Check sheet for the modelled part. Datum: model origin and axes. Units: mm. A direction names the side the tool comes from. Give positions to 0.01 mm unless a question says otherwise; leave off trailing zeros. Order: outer loops, then holes, each group sorted by start corner. A loop starts at its lowest first (then second) coordinate and runs counter-clockwise, first axis right, second up. Notation, with made-up numbers: M 26.25,36 L 68.25,36 A9 ccw 68.25,43 Z; hole C 25.25,-21.5 d4. An arc over 180 degrees is marked long. Answer in a Markdown table with one row per item. Add a question column.
Autodesk Inventor part; units mm, degrees
ref_plane "Work Plane1" through (91.4, 0, 0) normal (1, 0, 0) x (0, 0, -1)
ref_plane "YZ Plane" through (0, 0, 0) normal (1, 0, 0) x (0, 1, 0)
ref_plane "XZ Plane" through (0, 0, 0) normal (0, 1, 0) x (-1, 0, 0)
sketch "Sketch1" plane through (0, 0, 0) normal (1, 0, 0) x (0, 1, 0)
  line L0 (0, 0) -> (95, 0)
  line L1 (95, 0) -> (95, -67.5)
  line L2 (0, 0) -> (0, -80)
  line L3 (0, -80) -> (62.9325, -5)
  line L4 (0, -80) -> (117.6394, -80) construction
  line L5 (67.5, -95) -> (95, -67.5)
  line L6 (90, -5) -> (90, -67.5)
  line L7 (62.5, -95) -> (67.5, -95)
  line L8 (62.5, -95) -> (90, -67.5)
  line L9 (57.9325, -5) -> (5, -68.9585)
  line L10 (5, -5) -> (5, -68.9585)
  line L11 (90, -5) -> (62.9325, -5)
  line L12 (57.9325, -5) -> (5, -5)
  point P0 (0, -75)
  dimension "d0" = 95
  dimension "d2" = 80
  dimension "d5" = 50
  dimension "d22" = 5
  dimension "d23" = 5
  dimension "d24" = 27.5
  dimension "d27" = 5
  dimension "d28" = 5
  dimension "d29" = 5
  dimension "d30" = 50.389
  dimension "d31" = 95
  dimension "d32" = 67.5
  dimension "d34" = 68.9585
  dimension "d35" = 5
  dimension "d36" = 27.5
extrude "Extrusion1" add sketch "Sketch1" along normal blind 177.8
sketch "Sketch3" plane through (177.8, 0, 0) normal (1, 0, 0) x (0, 0, -1)
  line L0 (0, 95) -> (0, 0)
  line L1 (67.5, 95) -> (0, 95)
  line L2 (95, 67.5) -> (67.5, 95)
  line L3 (0, 0) -> (80, 0)
  line L4 (0, 95) -> (67.5, 95)
  line L5 (80, 0) -> (0, 0)
  line L6 (0, 0) -> (0, 95)
  line L7 (80, 0) -> (5, 62.9325)
  line L8 (80, 0) -> (53.1884, 22.4976)
  line L9 (53.1884, 22.4976) -> (80, 62.5)
  line L10 (95, 62.5) -> (67.5, 90)
  line L11 (95, 62.5) -> (80, 62.5)
  line L12 (67.5, 95) -> (95, 67.5)
  line L13 (67.5, 95) -> (95, 67.5)
  line L14 (95, 67.5) -> (95, 62.5)
  line L15 (95, 62.5) -> (95, 67.5)
  dimension "d37" = 35
  dimension "d39" = 15
  dimension "d40" = 40.0024
extrude "Extrusion2" add sketch "Sketch3" along normal blind 5
ref_plane "Work Plane1" through (91.4, 0, 0) normal (1, 0, 0) x (0, 0, -1)
mirror "Mirror1" about plane through (91.4, 0, 0) normal (1, 0, 0) of "Extrusion2"
properties part number "plowV3"
Q1. Go/stop test with flat-tipped pins: pin 1 (3 mm diameter, centred on x = 20.5, y = 43, fed in from +Z); pin 2 (6 mm diameter, centred on x = 133, y = 76.5, fed in from -Z); pin 3 (4 mm diameter, centred on x = 3.5, z = -86.5, fed in from -Y). Record where each tip stops, or that it passes through.
Q2. Draft check along X on faces 1 (the flat face through (0, 47, -36)), 2 (the flat face through (90, 0, -39)), 3 (the flat face through (90, 5, -37)), 4 (the flat face through (177.8, 64, -49)). Enter one of: pulls with the +X half, pulls with the -X half, needs draft (parallel to the pull), parting line crosses it, or undercut.
Q3. Thickness scan on probe 1 along X at (y, z) = (13.5, -43); probe 2 along Y at (x, z) = (135, -25); probe 3 along Y at (x, z) = (49, -6). Record the ranges inside material, lowest first.
Q4. Cross-section at B-B (z = -58.5). Record the boundary of the cut face in (x, y).
Q5. Tool access check on faces 5 (the flat face through (3, 62.5, -87)), 6 (the flat face through (90.19, 31.84, -36.53)), 7 (the flat face through (180.265, 42.219, -66.407)). Record the directions out of +Z, -Z, +X, -X, +Y, -Y that give a thin tool (end or side, any length) a straight path to the whole face; none if there is none.
Q6. Cross-section at A-A (y = 85). Record the boundary of the cut face in (x, z).
Q7. Cross-section at D-D (z = -84.5). Record the boundary of the cut face in (x, y).
Q8. Cross-section at C-C (x = 86). Record the boundary of the cut face in (y, z).
Values follow:
| question | item | result |
|---|---|---|
| 1 | pin 1 | z = 0 |
| 1 | pin 2 | z = -89 |
| 1 | pin 3 | y = 62.5 |
| 2 | face 1 | pulls with the -X half |
| 2 | face 2 | needs draft |
| 2 | face 3 | undercut |
| 2 | face 4 | undercut |
| 3 | probe 1 | 0 to 5, 177.8 to 182.8 |
| 3 | probe 2 | 0 to 5, 41.38 to 46.15, 90 to 95 |
| 3 | probe 3 | 0 to 5, 57.1 to 62.09, 90 to 95 |
| 4 | outline | M 0,0 L 182.8,0 L 182.8,18.04 L 0,18.04 Z; M 0,30.42 L 5,30.42 L 5,90 L 177.8,90 L 177.8,30.42 L 182.8,30.42 L 182.8,95 L 0,95 Z; hole M 5,5 L 177.8,5 L 177.8,13.66 L 5,13.66 Z |
| 5 | face 5 | -Z, +X, -X, -Y |
| 5 | face 6 | none |
| 5 | face 7 | -Z, +X, -X |
| 6 | outline | M 0,-77.5 L 182.8,-77.5 L 182.8,0 L 0,0 Z; hole M 5,-72.5 L 177.8,-72.5 L 177.8,-5 L 5,-5 Z |
| 7 | outline | M 0,62.5 L 5,62.5 L 5,73 L 177.8,73 L 177.8,62.5 L 182.8,62.5 L 182.8,78 L 0,78 Z |
| 8 | outline | M 0,-80 L 62.93,-5 L 90,-5 L 90,-67.5 L 62.5,-95 L 67.5,-95 L 95,-67.5 L 95,0 L 0,0 Z; hole M 5,-68.96 L 57.93,-5 L 5,-5 Z |
